```python
from build123d import *

# Parameters (mm, degrees)
F0_W     = 25
F0_H     = 114
F1_DEPTH = 3
F2_W     = 21
F2_H     = 113
F3_DEPTH = 2
F4_W     = 1
F4_H     = 1
F5_DEPTH = 113
F6_DEPTH = 1
F7_R     = 0.5


with BuildPart() as f1:
    # F0 (on Top) → F1 (new body)
    with BuildSketch(Plane.XY):
        Rectangle(F0_W, F0_H)
    extrude(amount=F1_DEPTH)

    # F2 (on face) → F3 (cut)
    with BuildSketch(Plane.XY.offset(3)):
        with Locations((0, 0.5)):
            Rectangle(F2_W, F2_H)
    extrude(amount=-F3_DEPTH, mode=Mode.SUBTRACT)

    # F4 (on face) → F5 (cut)
    with BuildSketch(Plane(origin=(0, 57, 0), x_dir=(-1, 0, 0), z_dir=(0, 1, 0))):
        with Locations((11, 1.5)):
            Rectangle(F4_W, F4_H)
    extrude(amount=-F5_DEPTH, mode=Mode.SUBTRACT)

    # F6 (add): a face of the model
    f6_faces = [f1.faces().sort_by_distance(p)[0] for p in [
        (0.34375, 57, 0.84375),
    ]]
    extrude(f6_faces, amount=F6_DEPTH)

    # F7
    f7_edges = [f1.edges().sort_by_distance(p)[0] for p in [
        (12.5, 0.5, 0),
        (12.5, 0.5, 3),
        (0, -57, 3),
        (0, -57, 0),
        (-12.5, 0.5, 3),
        (-12.5, 0.5, 0),
    ]]
    fillet(f7_edges, radius=F7_R)


solid = f1.part
```
For this review, take the finished solid that the model builds, in its own axes (mm). A direction names the side the tool comes from. Give positions to 0.01 mm unless a question says otherwise; leave off trailing zeros. Loops run counter-clockwise (first coordinate to the right, second up) from the corner with the lowest first, then second, coordinate; pieces in that order, holes last. Notation, with made-up numbers: M 19,16.5 L 33,16.5 A24 ccw 33,54.5 Z; hole C 88,21 d8. An arc over 180 degrees is marked long. One line per item, written item: value. Start each with the question number.
Q1. Add section A-A (z = 1.55). Give the boundary of the cut face in (x, y).
Q2. Add section B-B (x = 2). Give the boundary of the cut face in (y, z).
Q3. For L1, parallel to X at y = 48.5, z = 1.15; L2, parallel to Z at x = -1.25, y = -24.5; L3, parallel to Y at x = 0.25, z = 2.3, list the stretches that pass through material, from the lowest coordinate up.
Q4. Add section C-C (y = -21.5). Give the boundary of the cut face in (x, z).
Q5. Clearance check with a flat-ended pin moving along its axis: pin 1 Ø8 at (x, y) = (-1.5, -23) entering from +Z. State where the tip first meets the part, or that it passes through.
Q6. Machinability: for faces 4 (the face through (-12.5, 0, 1)), 5 (the face through (10.5, 0, 2)), which of the approach directions +Z, -Z, +X, -X, +Y, -Y give a long, thin tool a straight path to every point of the face, cutting with its end or side? Answer none if there is none.
Q7. Draft analysis for pull direction X (two halves, no side actions). For faces 1 (the face through (-1, 0, 1)), 2 (the face through (-11, 0, 3)), 3 (the face through (12.5, 0, 1)), state which applies: released by +X, released by -X, zero draft, split by the parting line, or undercut.
Reply:
1. outline: M -12.5,-57 L 12.5,-57 L 12.5,58 L 10.5,58 L 10.5,-56 L -11.5,-56 L -11.5,58 L -12.5,58 Z
2. outline: M -57,0.5 A0.5 ccw -56.5,0 L 58,0 L 58,1 L -56,1 L -56,3 L -56.5,3 A0.5 ccw -57,2.5 Z
3. L1: -12.5 to -11.5, 10.5 to 12.5
3. L2: 0 to 1
3. L3: -57 to -56
4. outline: M -12.5,0.5 A0.5 ccw -12,0 L 12,0 A0.5 ccw 12.5,0.5 L 12.5,2.5 A0.5 ccw 12,3 L 10.5,3 L 10.5,1 L -11.5,1 L -11.5,2 L -10.5,2 L -10.5,3 L -12,3 A0.5 ccw -12.5,2.5 Z
5. pin 1: z = 1
6. face 4: +Z, -Z, -X, +Y, -Y
6. face 5: +Z, +Y
7. face 1: undercut
7. face 2: zero draft
7. face 3: released by +X
